Geometry: final body of the model. Coordinates: model frame, mm. Face numbers are marked on the shaded views. A direction names the side the tool comes from. Give positions to 0.01 mm unless a question says otherwise; leave off trailing zeros. Order: outer loops, then holes, each group sorted by start corner. A loop starts at its lowest first (then second) coordinate and runs counter-clockwise, first axis right, second up. Notation, with made-up numbers: (-25, 69.5) - (-15, 69.5) arc R14 cw to (-15, 92.5) - close; hole circle Ø8 at (22.25, 82). An arc over 180 degrees is marked (long way). One line per question, with ' | ' between items. Start each with the question number.
from build123d import *

# Parameters (mm, degrees)
F0_W     = 36.5
F0_H     = 36.5
F0_R     = 1.75
F1_DEPTH = 0.2
F2_W     = 36.5
F2_H     = 36.5
F2_R     = 1.75
F2_R_2   = 3
F3_DEPTH = 1.8
F4_W     = 17.5
F4_H     = 36.5
F4_R     = 1.75
F4_R_2   = 3
F5_DEPTH = 0.4
F6_R     = 2.5


with BuildPart() as f1:
    # F0 (on Top) → F1 (new body)
    with BuildSketch(Plane.XY):
        with Locations((-17.7327652574, -14.8268600106)):
            Rectangle(F0_W, F0_H)
        with Locations((-32.9827652574, -30.0768600106)):
            Circle(F0_R, mode=Mode.SUBTRACT)
        with Locations((-2.4827652574, -30.0768600106)):
            Circle(F0_R, mode=Mode.SUBTRACT)
        with Locations((-32.9827652574, 0.4231399894)):
            Circle(F0_R, mode=Mode.SUBTRACT)
        with Locations((-2.4827652574, 0.4231399894)):
            Circle(F0_R, mode=Mode.SUBTRACT)
    extrude(amount=F1_DEPTH)

    # F2 (on face) → F3 (join)
    with BuildSketch(Plane.XY.offset(0.2)):
        with Locations((-17.7327652574, -14.8268600106)):
            Rectangle(F2_W, F2_H)
        with Locations((-32.9827652574, -30.0768600106)):
            Circle(F2_R, mode=Mode.SUBTRACT)
        with Locations((-25.8577652574, -20.8268600106)):
            Circle(F2_R_2, mode=Mode.SUBTRACT)
        with Locations((-2.4827652574, -30.0768600106)):
            Circle(F2_R, mode=Mode.SUBTRACT)
        with Locations((-9.6077652574, -20.8268600106)):
            Circle(F2_R_2, mode=Mode.SUBTRACT)
        with Locations((-25.8577652574, -8.8268600106)):
            Circle(F2_R_2, mode=Mode.SUBTRACT)
        with Locations((-32.9827652574, 0.4231399894)):
            Circle(F2_R, mode=Mode.SUBTRACT)
        with Locations((-9.6077652574, -8.8268600106)):
            Circle(F2_R_2, mode=Mode.SUBTRACT)
        with Locations((-2.4827652574, 0.4231399894)):
            Circle(F2_R, mode=Mode.SUBTRACT)
    extrude(amount=F3_DEPTH)

    # F4 (on face) → F5 (join)
    with BuildSketch(Plane.XY.offset(2)):
        with Locations((-8.2327652574, -14.8268600106)):
            Rectangle(F4_W, F4_H)
        with Locations((-2.4827652574, -30.0768600106)):
            Circle(F4_R, mode=Mode.SUBTRACT)
        with Locations((-9.6077652574, -20.8268600106)):
            Circle(F4_R_2, mode=Mode.SUBTRACT)
        with Locations((-9.6077652574, -8.8268600106)):
            Circle(F4_R_2, mode=Mode.SUBTRACT)
        with Locations((-2.4827652574, 0.4231399894)):
            Circle(F4_R, mode=Mode.SUBTRACT)
    extrude(amount=F5_DEPTH)

    # F6
    f6_edges = [f1.edges().sort_by_distance(p)[0] for p in [
        (-35.982765, 3.42314, 1),
        (-35.982765, -33.07686, 1),
        (0.517235, -33.07686, 1.2),
        (0.517235, 3.42314, 1.2),
    ]]
    fillet(f6_edges, radius=F6_R)


solid = f1.part
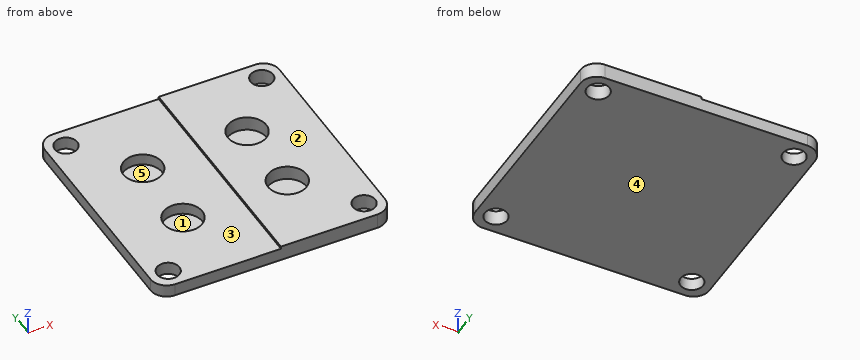
(1) Cut plane A-A, the plane z = 1.5. Give the number of separate pieces and of enclosed holes in the cut face, plus the area to 3 significant figures.
(2) Cut plane C-C, the plane y = 0. Return the cut outline in (x, z).
(3) Material intervals for line 1 along Y through (x, z) = (-9.5, 0.85); line 2 along X through (y, z) = (-30, 0.7); line 3 along X through (y, z) = (-11, 0.85), sorted ascending. Write a range as from..to.
(4) Pull-direction query (X, two-part tool) for the marked faces 4 and 5; classes: +X half, -X half, draft (parallel to the pull), parting line (faces both ways), or undercut.
(5) Cut plane D-D, the plane x = -28. Return the cut outline in (y, z).
(6) Cut plane B-B, the plane x = -33. Return the cut outline in (y, z), plus the area to 3 significant figures.
(7) Access query for the marked faces 1, 2 and 3. Directions: +Z, -Z, +X, -X, +Y, -Y. A direction counts if a zero-diameter tool reaches every point of the face in a straight line with its end or side. Return the directions, or none.
(8) Contact query for flat-ended pins moving along their axis: P1, Ø8, axis at x = -31, y = -26.5, coming from the +Z side; P2, Ø3, axis at x = -26, y = -19.5, coming from the +Z side; P3, Ø5.5, axis at x = -2.48, y = -30.08, coming from the +Z side; P4, Ø3, axis at x = -32.98, y = 0.42, coming from the +Z side. Output: stop coordinate, or through.
Results are:
1) separate pieces: 1 | enclosed holes: 8 | area: 1,180 mm2
2) outline: (-35.98, 0) - (-34.68, 0) - (-34.68, 2) - (-35.98, 2) - close; (-31.28, 0) - (-4.18, 0) - (-4.18, 2.4) - (-16.98, 2.4) - (-16.98, 2) - (-31.28, 2) - close; (-0.78, 0) - (0.52, 0) - (0.52, 2.4) - (-0.78, 2.4) - close
3) line 1: -33.08..-23.82, -17.83..-11.82, -5.83..3.42 | line 2: -35.98..-34.73, -31.23..-4.23, -0.73..0.52 | line 3: -35.98..-27.93, -23.79..-11.68, -7.54..0.52
4) face 4: draft | face 5: undercut
5) outline: (-33.08, 0) - (3.42, 0) - (3.42, 2) - (-6.73, 2) - (-6.73, 0.2) - (-10.93, 0.2) - (-10.93, 2) - (-18.73, 2) - (-18.73, 0.2) - (-22.93, 0.2) - (-22.93, 2) - (-33.08, 2) - close
6) outline: (-33.08, 0) - (-31.83, 0) - (-31.83, 2) - (-33.08, 2) - close; (-28.33, 0) - (-1.33, 0) - (-1.33, 2) - (-28.33, 2) - close; (2.17, 0) - (3.42, 0) - (3.42, 2) - (2.17, 2) - close | area: 59.0 mm2
7) face 1: +Z | face 2: +Z, +X, -X, +Y, -Y | face 3: +Z, -X, +Y, -Y
8) P1: z = 2 | P2: z = 0.2 | P3: z = 2.4 | P4: through
